```python
from build123d import *

# Parameters (mm, degrees)
SKETCH1_R          = 1.25
EXTRUDE1_DEPTH     = 0.75
FILLET1_R          = 1.48
CUT_EXTRUDE1_DEPTH = 2.5
FILLET2_R          = 2


with BuildPart() as part:
    # Sketch1 → Extrude1 (new body, symmetric)
    with BuildSketch(Plane(origin=(0, 0, 0), x_dir=(0, 0, -1), z_dir=(1, 0, 0))):
        with BuildLine():
            Line((-0.258295615, 14.797745888), (-0.349048129, 19.996953903))
            ThreePointArc((-0.349048129, 19.996953903), (-4.163801356, 19.561767769), (-7.825100504, 18.40564593))
            Line((-7.825100504, 18.40564593), (-8.717280741, 14.827306447))
            ThreePointArc((-8.717280741, 14.827306447), (0, -18.4), (8.717280741, 14.827306447))
            Line((8.717280741, 14.827306447), (7.825100504, 18.40564593))
            ThreePointArc((7.825100504, 18.40564593), (4.163801356, 19.561767769), (0.349048129, 19.996953903))
            Line((0.349048129, 19.996953903), (0.258295615, 14.797745888))
            ThreePointArc((0.258295615, 14.797745888), (0, -14.8), (-0.258295615, 14.797745888))
        make_face()
        with Locations((-3.85879125, 17.335295056)):
            Circle(SKETCH1_R, mode=Mode.SUBTRACT)
        with Locations((3.85879125, 17.335295056)):
            Circle(SKETCH1_R, mode=Mode.SUBTRACT)
    extrude(amount=EXTRUDE1_DEPTH, both=True)

    # Fillet1
    fillet1_edges = [part.edges().sort_by_distance(p)[0] for p in [
        (0, 18.40564593, -7.825100504),
        (0, 14.827306447, -8.717280741),
        (0, 14.827306447, 8.717280741),
        (0, 18.40564593, 7.825100504),
    ]]
    fillet(fillet1_edges, radius=FILLET1_R)

    # Sketch3 → Cut-Extrude1 (cut, through all)
    with BuildSketch(Plane(origin=(0.75, 0, 0), x_dir=(0, 0, -1), z_dir=(1, 0, 0))):
        Polygon((0, 0), (0, 37.659404293), (33.944851403, 0), align=None)
    extrude(amount=-CUT_EXTRUDE1_DEPTH, mode=Mode.SUBTRACT)

    # Fillet2
    fillet2_edges = [part.edges().sort_by_distance(p)[0] for p in [
        (0, 0, -14.8),
    ]]
    fillet(fillet2_edges, radius=FILLET2_R)


solid = part.part
```
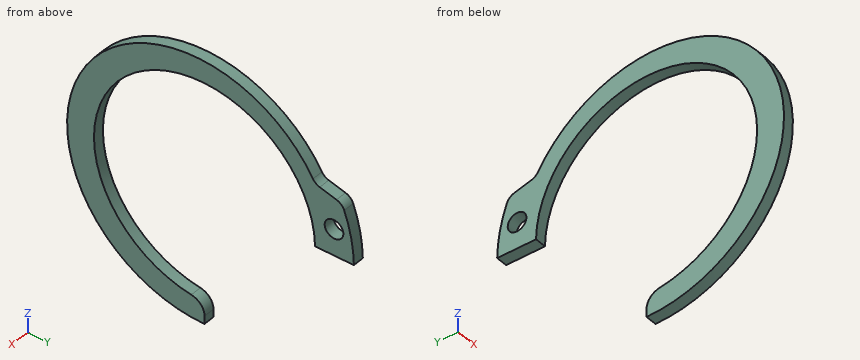
Check sheet for the modelled part. Datum: model origin and axes. Units: mm. Give positions to 0.01 mm unless a question says otherwise; leave off trailing zeros. Write each loop counter-clockwise with the first axis right and the second up, starting at its lowest first coordinate (ties: lowest second). Pieces come first, ordered by that corner, then holes. Notation, with made-up numbers: (9, 11.25) -> (41, 11.25) arc R23 cw to (41, 26.25) -> close; hole circle Ø1 at (44.25, 24). An arc over 180 degrees is marked (long way). Use CSV: the item, a comma, the result in double quotes. Start each with the question number.
Q1. Scan lines: line 1 along Y through (x, z) = (0.3, 0); line 2 along Z through (x, y) = (-0.35, -3.5); line 3 along Z through (x, y) = (-0.5, -0.5). Record each from-to range of solid material in increasing order.
Q2. Cross-section at C-C on y = 3. Enter the section's corners in (x, z).
Q3. Cross-section at A-A on y = -5. Enter the section's corners in (x, z).
Q4. Cross-section at B-B on x = 0.25. Enter the section's corners in (y, z), and give its area (3 significant figures).
Q5. Cross-section at D-D on y = 8.5. Enter the section's corners in (x, z).
Q6. Depth check by flat-ended pin: P1, Ø3, axis at y = 17.34, z = 3.86, coming from the -X side. Enter the tip coordinate at first touch or a pass-through.
Working result:
1,line 1,"y = -18.4 to -14.8"
1,line 2,"z = -17.53 to -14.38, 14.38 to 17.53"
1,line 3,"z = -17.76 to -15.36, 14.79 to 17.76"
2,outline,"(-0.75, 14.49) -> (0.75, 14.49) -> (0.75, 17.38) -> (-0.75, 17.38) -> close"
3,outline,"(-0.75, -17.21) -> (0.75, -17.21) -> (0.75, -13.93) -> (-0.75, -13.93) -> close; (-0.75, 13.93) -> (0.75, 13.93) -> (0.75, 17.21) -> (-0.75, 17.21) -> close"
4,outline,"(-1.76, -14.69) arc R14.8 cw (long way) to (14.8, 0.26) -> (20, 0.35) arc R20 ccw to (18.7, 7.1) arc R1.48 ccw to (17.67, 8.01) -> (15.43, 8.57) arc R1.48 cw to (14.53, 9.23) arc R17.76 ccw (long way) to (0, -17.75) -> (0, -16.68) arc R2 ccw to start; hole circle Ø2.5 at (17.34, 3.86)"
4,area,"256 mm^2"
5,outline,"(-0.75, 12.12) -> (0.75, 12.12) -> (0.75, 15.22) -> (-0.75, 15.22) -> close"
6,P1,"stops at x = -0.75"
